from build123d import *

# Parameters (mm, degrees)
SKETCH_1_W          = 33
SKETCH_1_H          = 39
EXTRUDE_1_DEPTH     = 1
SKETCH_2_R          = 12.5
EXTRUDE_2_DEPTH     = 6.5
EXTRUDE_3_DEPTH     = 10
SKETCH_4_R          = 2.3
EXTRUDE_4_DEPTH     = 20
SKETCH_5_OUTSIDE_W  = 62.518
SKETCH_5_OUTSIDE_H  = 57.518
SKETCH_5_OUTSIDE_R  = 12.5
CUT_EXTRUDE_1_DEPTH = 5


with BuildPart() as part:
    # Sketch 1 → Extrude 1 (new body)
    with BuildSketch(Plane(origin=(0, 0, 0), x_dir=(1, 0, 0), z_dir=(0, 1, 0))):
        Rectangle(SKETCH_1_W, SKETCH_1_H)
    extrude(amount=EXTRUDE_1_DEPTH)



with BuildPart() as body_2:
    # Sketch 2 → Extrude 2 (new, symmetric)
    with BuildSketch(Plane.XY):
        with Locations(Location((-15, -24.5, 0), (0, 0, 180))):
            Circle(SKETCH_2_R)
    extrude(amount=EXTRUDE_2_DEPTH, both=True)


with BuildPart() as part_1:
    add(part.part)

    add(body_2.part)  # Extrude 3 merges body 2
    # Sketch 3 → Extrude 3 (add, symmetric)
    with BuildSketch(Plane.XY):
        with BuildLine():
            Line((-12.5, 0), (-11.111866784, -6.574487566))
            Line((-11.111866784, -6.574487566), (-15, -12))
            ThreePointArc((-15, -12), (-9.487173184, -13.281321802), (-5.104539199, -16.86260152))
            Line((-5.104539199, -16.86260152), (12.5, 0))
            Line((12.5, 0), (-12.5, 0))
        make_face()
    extrude(amount=EXTRUDE_3_DEPTH, both=True)

    # Sketch 4 → Extrude 4 (add)
    with BuildSketch(Plane(origin=(0, 1, 0), x_dir=(1, 0, 0), z_dir=(0, 1, 0))):
        with Locations(Location((-12, 15, 0), (0, 0, 270))):
            Circle(SKETCH_4_R)
        with Locations(Location((12, 15, 0), (0, 0, 270))):
            Circle(SKETCH_4_R)
        with Locations(Location((-12, -15, 0), (0, 0, 270))):
            Circle(SKETCH_4_R)
        with Locations(Location((12, -15, 0), (0, 0, 270))):
            Circle(SKETCH_4_R)
    extrude(amount=EXTRUDE_4_DEPTH)

    # Sketch 5 outside → Cut-Extrude 1 (cut)
    with BuildSketch(Plane.XZ):
        with Locations((-5.5, 0)):
            Rectangle(SKETCH_5_OUTSIDE_W, SKETCH_5_OUTSIDE_H)
        Circle(SKETCH_5_OUTSIDE_R, mode=Mode.SUBTRACT)
    extrude(amount=CUT_EXTRUDE_1_DEPTH, mode=Mode.SUBTRACT)


solid = part_1.part
Read the model definition and answer for the solid it produces. Units are mm, in the model's axes. A direction names the side the tool comes from. Coordinates: 2 decimals unless noted, no trailing zeros. Loops run counter-clockwise (first coordinate to the right, second up) from the corner with the lowest first, then second, coordinate; pieces in that order, holes last. Notation, with made-up numbers: (75, -37.5) - (125, -37.5) arc R23 cw to (125, -24.5) - close; hole circle Ø4 at (19.5, -20.75). An arc over 180 degrees is marked (long way). Answer in a Markdown table with one row per item.
Q1. The mould has two halves that part along Y. Classify faces 1 (the flat face through (-11.66, -3.97, 0.14)), 2 (the flat face through (12, 21, -15)), 3 (the flat face through (-15, -25, 6.5)): pulls with the +Y half, pulls with the -Y half, needs draft (parallel to the pull), parting line crosses it, or undercut.
Here are the results:
| item | result |
|---|---|
| face 1 | undercut |
| face 2 | pulls with the +Y half |
| face 3 | needs draft |
Q2. Find section D-D on y = -13.5. Write down the section's boundary in (x, z), plus the area to 3 significant figures.
Here are the results:
| item | result |
|---|---|
| outline | (-20.94, -6.5) - (-9.06, -6.5) - (-9.06, -10) - (-1.59, -10) - (-1.59, 10) - (-9.06, 10) - (-9.06, 6.5) - (-20.94, 6.5) - close |
| area | 304 mm^2 |
Q3. Straight lines are drawn through the part: line 1 along X through (y, z) = (6.5, 15); line 2 along Z through (x, y) = (-11.5, -26.5); line 3 along Y through (x, z) = (-1.5, -14). For each, find the intervals that lie inside material, in ascending order. Write a range as [from, to].
Here are the results:
| item | result |
|---|---|
| line 1 | x = [-14.3, -9.7], [9.7, 14.3] |
| line 2 | z = [-6.5, 6.5] |
| line 3 | y = [0, 1] |
Q4. Given P1, Ø18.5, axis at x = -7, y = -11, coming from the +Z side; P2, Ø16.5, axis at x = -5.5, z = -5, coming from the -Y side; P3, Ø8, axis at x = 6.5, y = -10, coming from the -Z side; P4, Ø8, axis at x = 5, y = 4, coming from the -Z side, each flat-ended and moving along its own axis, determine where each tip first touches the part or whether it passes through.
Here are the results:
| item | result |
|---|---|
| P1 | stops at z = 10 |
| P2 | stops at y = -36.94 |
| P3 | stops at z = -10 |
| P4 | stops at z = -19.5 |
Q5. Find section A-A on z = 15. Write down the section's boundary in (x, y), plus the area to 3 significant figures.
Here are the results:
| item | result |
|---|---|
| outline | (-16.5, 0) - (16.5, 0) - (16.5, 1) - (14.3, 1) - (14.3, 21) - (9.7, 21) - (9.7, 1) - (-9.7, 1) - (-9.7, 21) - (-14.3, 21) - (-14.3, 1) - (-16.5, 1) - close |
| area | 217 mm^2 |
Q6. Find section B-B on y = 3. Write down the section's boundary in (x, z).
Here are the results:
| item | result |
|---|---|
| outline | circle Ø4.6 at (-12, -15); circle Ø4.6 at (-12, 15); circle Ø4.6 at (12, -15); circle Ø4.6 at (12, 15) |
Q7. For faces 4 (the cylindrical face through (-9.559, -13.246, 8.274)), 5 (the flat face through (0, 0, -13)), 6 (the cylindrical face through (-9.559, -13.246, -8.226)), determine the directions among +Z, -Z, +X, -X, +Y, -Y from which every point of the face is accessible in a straight line to the end or side of a thin tool.
Here are the results:
| item | result |
|---|---|
| face 4 | +Z, -X, -Y |
| face 5 | none |
| face 6 | -Z, -X, -Y |
Q8. Find section C-C on x = 4.5. Write down the section's boundary in (y, z), plus the area to 3 significant figures.
Here are the results:
| item | result |
|---|---|
| outline | (-7.66, -10) - (0, -10) - (0, -19.5) - (1, -19.5) - (1, 19.5) - (0, 19.5) - (0, 10) - (-7.66, 10) - close |
| area | 192 mm^2 |
